The model under review builds one solid part; all positions refer to its coordinate system, in mm. A direction names the side the tool comes from. Coordinates: 2 decimals unless noted, no trailing zeros. Write each loop counter-clockwise with the first axis right and the second up, starting at its lowest first coordinate (ties: lowest second). Pieces come first, ordered by that corner, then holes. Notation, with made-up numbers: M -23,-36 L -2,-36 A25 ccw -2,-23 Z; hole C 33,-33 d3. An arc over 180 degrees is marked long. Answer as a JSON object with one key per item and string values.
```python
from build123d import *

# Parameters (mm, degrees)
F2_R     = 25
F2_R_2   = 20
F3_DEPTH = 15
F4_DEPTH = 30
F5_R     = 12.7094
F6_DEPTH = 15


with BuildPart() as f3:
    # F2 (on Top) → F3 (new body)
    with BuildSketch(Plane.XY):
        Circle(F2_R)
        Circle(F2_R_2, mode=Mode.SUBTRACT)
    extrude(amount=F3_DEPTH)

    # F2 (on Top) → F4 (join)
    with BuildSketch(Plane.XY):
        Circle(F2_R_2)
    extrude(amount=F4_DEPTH)

    # F5 (on face) → F6 (cut)
    with BuildSketch(Plane.XY.offset(30)):
        Circle(F5_R)
    extrude(amount=-F6_DEPTH, mode=Mode.SUBTRACT)


solid = f3.part
```
(1) For faces 1 (the face through (0, -13, 30)), 2 (the face through (0, 0, 15)), list the 3-axis set-ups (+Z, -Z, +X, -X, +Y, -Y) from which the entire face can be reached by the end or side of a thin tool; tool diameter is ignored.
Results list:
{"face 1": "+Z, +X, -X, +Y, -Y", "face 2": "+Z"}
(2) Draft analysis for pull direction X (two halves, no side actions). For faces 3 (the face through (-2.755, -12.407, 22.605)), 4 (the face through (23.846, 7.509, 7.395)), 5 (the face through (0, 0, 0)), state which applies: released by +X, released by -X, zero draft, split by the parting line, or undercut.
Results list:
{"face 3": "undercut", "face 4": "split by the parting line", "face 5": "zero draft"}
(3) Wall thickness on line 1 along Y through (x, z) = (0, 21); line 2 along Z through (x, y) = (6, -19.5); line 3 along Y through (x, z) = (5, 23.5): over which ranges is each line inside the solid? List them lowest first. Write a range as from..to.
Results list:
{"line 1": "-20..-12.71, 12.71..20", "line 2": "0..15", "line 3": "-19.36..-11.68, 11.68..19.36"}
(4) Add section C-C on z = 27.25. Give the boundary of the cut face in (x, y).
Results list:
{"outline": "C 0,0 d40; hole C 0,0 d25.42"}
(5) Add section A-A on x = 0. Give the boundary of the cut face in (y, z).
Results list:
{"outline": "M -25,0 L 25,0 L 25,15 L 20,15 L 20,30 L 12.71,30 L 12.71,15 L -12.71,15 L -12.71,30 L -20,30 L -20,15 L -25,15 Z"}
(6) Add section D-D on x = -17. Give the boundary of the cut face in (y, z).
Results list:
{"outline": "M -18.33,0 L 18.33,0 L 18.33,15 L 10.54,15 L 10.54,30 L -10.54,30 L -10.54,15 L -18.33,15 Z"}
(7) For pin 1 Ø5 at (y, z) = (5.5, 11.5) entering from -X; pin 2 Ø10 at (x, z) = (-1.5, 13) entering from -Y; pin 3 Ø4 at (x, z) = (-5, 9.5) entering from -Y, all flat-tipped, find the tip position at first contact; note any pin that passes through.
Results list:
{"pin 1": "x = -24.82", "pin 2": "y = -25", "pin 3": "y = -24.82"}
